The listing builds one solid part. Answer for the finished solid, in the listing's coordinates (mm). A direction names the side the tool comes from. Coordinates: 2 decimals unless noted, no trailing zeros. Loops run counter-clockwise (first coordinate to the right, second up) from the corner with the lowest first, then second, coordinate; pieces in that order, holes last. Notation, with made-up numbers: (63, -17.75) -> (78, -17.75) arc R19 ccw to (78, 6.25) -> close; hole circle Ø10 at (0, 4). An arc over 180 degrees is marked (long way). Answer in a Markdown table with one row per item.
```python
from build123d import *

# Parameters (mm, degrees)
SKETCH1_W                     = 278.2
SKETCH1_H                     = 193.2
SHELL_BLOCK_DEPTH             = 27
SKETCH2_W                     = 273.2
SKETCH2_H                     = 185.8
FRONT_OPENING_DEPTH           = 1.5
SKETCH3_W                     = 273.2
SKETCH3_H                     = 188.2
DISPLAY_POCKET_DEPTH          = 22.5
SKETCH4_W                     = 3
SKETCH4_H                     = 56
VENT_SLOTS_DEPTH              = 4
SKETCH5_W                     = 58
SKETCH5_H                     = 16
CABLE_EXIT_X_SHORT_SIDE_DEPTH = 140.1
SKETCH6_R                     = 1.7
BOLT_HOLES_DEPTH              = 4
KEEP_ONE_HALF_X_DEPTH         = 172.491603293
KEEP_ONE_HALF_X_DEPTH_BACK    = 172.491603293
SKETCH7_W                     = 200
SKETCH7_H                     = 400
KEEP_ONE_QUARTER_Z_DEPTH      = 172.491603293
KEEP_ONE_QUARTER_Z_DEPTH_BACK = 172.491603293
SKETCH8_W                     = 400
SKETCH8_H                     = 200


with BuildPart() as part:
    # Sketch1 → Shell Block (new body)
    with BuildSketch(Plane(origin=(0, 0, 0), x_dir=(1, 0, 0), z_dir=(0, 1, 0))):
        Rectangle(SKETCH1_W, SKETCH1_H)
    extrude(amount=SHELL_BLOCK_DEPTH)

    # Sketch2 → Front Opening (cut)
    with BuildSketch(Plane(origin=(0, 27, 0), x_dir=(1, 0, 0), z_dir=(0, 1, 0))):
        Rectangle(SKETCH2_W, SKETCH2_H)
    extrude(amount=-FRONT_OPENING_DEPTH, mode=Mode.SUBTRACT)

    # Sketch3 → Display Pocket (cut)
    with BuildSketch(Plane(origin=(0, 25.5, 0), x_dir=(1, 0, 0), z_dir=(0, 1, 0))):
        Rectangle(SKETCH3_W, SKETCH3_H)
    extrude(amount=-DISPLAY_POCKET_DEPTH, mode=Mode.SUBTRACT)

    # Sketch4 → Vent Slots (cut)
    with BuildSketch(Plane(origin=(0, 3, 0), x_dir=(1, 0, 0), z_dir=(0, 1, 0))):
        with Locations((-67.5, 56)):
            Rectangle(SKETCH4_W, SKETCH4_H)
        with Locations((-67.5, -56)):
            Rectangle(SKETCH4_W, SKETCH4_H)
        with Locations((-75.5, 56)):
            Rectangle(SKETCH4_W, SKETCH4_H)
        with Locations((-75.5, -56)):
            Rectangle(SKETCH4_W, SKETCH4_H)
        with Locations((-83.5, 56)):
            Rectangle(SKETCH4_W, SKETCH4_H)
        with Locations((-83.5, -56)):
            Rectangle(SKETCH4_W, SKETCH4_H)
        with Locations((-91.5, 56)):
            Rectangle(SKETCH4_W, SKETCH4_H)
        with Locations((-91.5, -56)):
            Rectangle(SKETCH4_W, SKETCH4_H)
        with Locations((-99.5, 56)):
            Rectangle(SKETCH4_W, SKETCH4_H)
        with Locations((-99.5, -56)):
            Rectangle(SKETCH4_W, SKETCH4_H)
        with Locations((-107.5, 56)):
            Rectangle(SKETCH4_W, SKETCH4_H)
        with Locations((-107.5, -56)):
            Rectangle(SKETCH4_W, SKETCH4_H)
        with Locations((-115.5, 56)):
            Rectangle(SKETCH4_W, SKETCH4_H)
        with Locations((-115.5, -56)):
            Rectangle(SKETCH4_W, SKETCH4_H)
        with Locations((-123.5, 56)):
            Rectangle(SKETCH4_W, SKETCH4_H)
        with Locations((-123.5, -56)):
            Rectangle(SKETCH4_W, SKETCH4_H)
    extrude(amount=-VENT_SLOTS_DEPTH, mode=Mode.SUBTRACT)

    # Sketch5 → Cable Exit (-X short side) (cut)
    with BuildSketch(Plane(origin=(0, 0, 0), x_dir=(0, 0, -1), z_dir=(1, 0, 0))):
        with Locations((0, 13)):
            Rectangle(SKETCH5_W, SKETCH5_H)
    extrude(amount=-CABLE_EXIT_X_SHORT_SIDE_DEPTH, mode=Mode.SUBTRACT)

    # Sketch6 → Bolt Holes (cut)
    with BuildSketch(Plane(origin=(0, 3, 0), x_dir=(1, 0, 0), z_dir=(0, 1, 0))):
        with Locations(Location((-40, -45, 0), (0, 0, 270))):
            Circle(SKETCH6_R)
        with Locations(Location((-40, 45, 0), (0, 0, 270))):
            Circle(SKETCH6_R)
        with Locations(Location((40, -45, 0), (0, 0, 270))):
            Circle(SKETCH6_R)
        with Locations(Location((40, 45, 0), (0, 0, 270))):
            Circle(SKETCH6_R)
        with Locations(Location((-52, -15, 0), (0, 0, 270))):
            Circle(SKETCH6_R)
        with Locations(Location((-52, 15, 0), (0, 0, 270))):
            Circle(SKETCH6_R)
        with Locations(Location((52, -15, 0), (0, 0, 270))):
            Circle(SKETCH6_R)
        with Locations(Location((52, 15, 0), (0, 0, 270))):
            Circle(SKETCH6_R)
        with Locations(Location((-12, -82, 0), (0, 0, 270))):
            Circle(SKETCH6_R)
        with Locations(Location((-12, 82, 0), (0, 0, 270))):
            Circle(SKETCH6_R)
        with Locations(Location((12, -82, 0), (0, 0, 270))):
            Circle(SKETCH6_R)
        with Locations(Location((12, 82, 0), (0, 0, 270))):
            Circle(SKETCH6_R)
        with Locations(Location((-124, -12, 0), (0, 0, 270))):
            Circle(SKETCH6_R)
        with Locations(Location((-124, 12, 0), (0, 0, 270))):
            Circle(SKETCH6_R)
        with Locations(Location((124, -12, 0), (0, 0, 270))):
            Circle(SKETCH6_R)
        with Locations(Location((124, 12, 0), (0, 0, 270))):
            Circle(SKETCH6_R)
    extrude(amount=-BOLT_HOLES_DEPTH, mode=Mode.SUBTRACT)

    # Sketch7 → Keep one half (X) (cut, two sides: drawn at the far end of the back side and taken through both)
    with BuildSketch(Plane(origin=(0, 0, 0), x_dir=(1, 0, 0), z_dir=(0, 1, 0)).offset(-KEEP_ONE_HALF_X_DEPTH_BACK)):
        with Locations((-100, 0)):
            Rectangle(SKETCH7_W, SKETCH7_H)
    extrude(amount=KEEP_ONE_HALF_X_DEPTH + KEEP_ONE_HALF_X_DEPTH_BACK, mode=Mode.SUBTRACT)

    # Sketch8 → Keep one quarter (Z) (cut, two sides: drawn at the far end of the back side and taken through both)
    with BuildSketch(Plane(origin=(0, 0, 0), x_dir=(1, 0, 0), z_dir=(0, 1, 0)).offset(-KEEP_ONE_QUARTER_Z_DEPTH_BACK)):
        with Locations((0, -100)):
            Rectangle(SKETCH8_W, SKETCH8_H)
    extrude(amount=KEEP_ONE_QUARTER_Z_DEPTH + KEEP_ONE_QUARTER_Z_DEPTH_BACK, mode=Mode.SUBTRACT)


solid = part.part
```
Item 1: A cutting plane is placed at D-D, the plane x = 45.5. Determine the outline of the cut face in (y, z).
Findings below:
| item | result |
|---|---|
| outline | (0, -96.6) -> (27, -96.6) -> (27, -92.9) -> (25.5, -92.9) -> (25.5, -94.1) -> (3, -94.1) -> (3, 0) -> (0, 0) -> close |
Item 2: A tool of negligible diameter and unlimited length cuts with its end or side. For faces 5 (the face through (67, 14, -94.1)), 6 (the face through (69, 13, -96.6)), from which of +Z, -Z, +X, -X, +Y, -Y can it reach the whole face along a straight path? Write none if from no direction.
Findings below:
| item | result |
|---|---|
| face 5 | +Z, -X |
| face 6 | -Z, +X, -X, +Y, -Y |
Item 3: A cutting plane is placed at B-B, the plane x = 12. Determine the outline of the cut face in (y, z).
Findings below:
| item | result |
|---|---|
| outline | (0, -96.6) -> (27, -96.6) -> (27, -92.9) -> (25.5, -92.9) -> (25.5, -94.1) -> (3, -94.1) -> (3, -83.7) -> (0, -83.7) -> close; (0, -80.3) -> (3, -80.3) -> (3, 0) -> (0, 0) -> close |
Item 4: Determine the mould class of faces 1 (the face through (69, 1, 0)), 2 (the face through (12.07, 1.52, -83.7)), 3 (the face through (124.51, 1.52, -10.38)), 4 (the face through (69, 0, -49)) for opening direction Z: +Z half, -Z half, draft (parallel to the pull), parting line (faces both ways), or undercut.
Findings below:
| item | result |
|---|---|
| face 1 | +Z half |
| face 2 | undercut |
| face 3 | undercut |
| face 4 | draft |
Item 5: A cutting plane is placed at A-A, the plane z = -45. Determine the outline of the cut face in (x, y), plus the area to 3 significant figures.
Findings below:
| item | result |
|---|---|
| outline | (0, 0) -> (38.3, 0) -> (38.3, 3) -> (0, 3) -> close; (41.7, 0) -> (139.1, 0) -> (139.1, 27) -> (136.6, 27) -> (136.6, 3) -> (41.7, 3) -> close |
| area | 467 mm2 |
Item 6: Flat-ended cylindrical pins translate along their axes: pin 1 Ø11 at (x, y) = (39.5, 19) entering from +Z; pin 2 Ø4.5 at (x, z) = (40, -45) entering from +Y; pin 3 Ø4 at (x, z) = (52, -15) entering from -Y; pin 4 Ø10 at (x, y) = (71.5, 21.5) entering from +Z. Find the tip coordinate at first contact, or state that the pin passes through.
Findings below:
| item | result |
|---|---|
| pin 1 | stops at z = -94.1 |
| pin 2 | stops at y = 3 |
| pin 3 | stops at y = 0 |
| pin 4 | stops at z = -92.9 |
Item 7: Find the intervals of material crossed by probe 1 along X at (y, z) = (0.8, -15); probe 2 along X at (y, z) = (1.25, -45); probe 3 along Y at (x, z) = (98.5, -45), in increasing order.
Findings below:
| item | result |
|---|---|
| probe 1 | x = 0 to 50.3, 53.7 to 139.1 |
| probe 2 | x = 0 to 38.3, 41.7 to 139.1 |
| probe 3 | y = 0 to 3 |
Item 8: A cutting plane is placed at C-C, the plane y = 19.5. Determine the outline of the cut face in (x, z), plus the area to 3 significant figures.
Findings below:
| item | result |
|---|---|
| outline | (0, -96.6) -> (139.1, -96.6) -> (139.1, 0) -> (136.6, 0) -> (136.6, -94.1) -> (0, -94.1) -> close |
| area | 583 mm2 |
